```python
from build123d import *

# Parameters (mm, degrees)
F0_W     = 170
F0_H     = 60
F1_DEPTH = 60
F2_R     = 20
F3_T     = -10
F4_SCALE = 1.2


with BuildPart() as f1:
    # F0 (on Top) → F1 (new body, symmetric)
    with BuildSketch(Plane.XY):
        Rectangle(F0_W, F0_H)
    extrude(amount=F1_DEPTH, both=True)

    # F2
    f2_edges = [f1.edges().sort_by_distance(p)[0] for p in [
        (-85, -30, 0),
        (-85, 30, 0),
        (85, -30, 0),
        (85, 30, 0),
        (0, 30, -60),
        (0, -30, -60),
        (-85, 0, -60),
        (85, 0, -60),
    ]]
    fillet(f2_edges, radius=F2_R)

    # F3
    f3_openings = [f1.faces().sort_by_distance(p)[0] for p in [
        (0, 0, 60),
    ]]
    offset(amount=F3_T, openings=f3_openings)


with BuildPart() as f1_1:
    # F4: moved
    add(f1.part.scale(F4_SCALE))


solid = f1_1.part
```
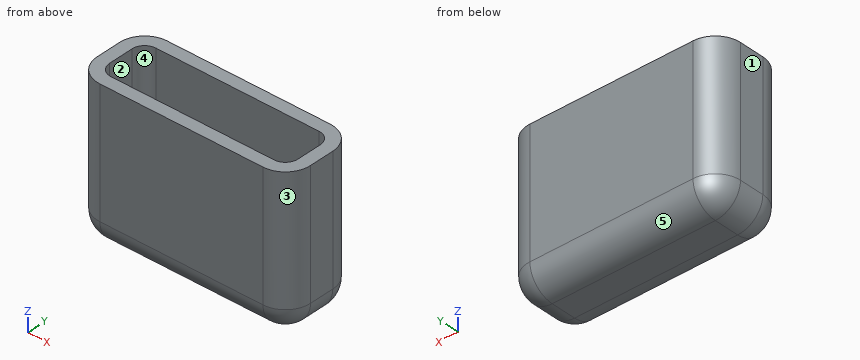
Here's how the part is built. I have some questions about the finished solid (model axes, mm). Face numbers are marked on the shaded views. A direction names the side the tool comes from. Round coordinates to 2 decimals unless told otherwise and drop trailing zeros. Order: outer loops, then holes, each group sorted by start corner. A loop starts at its lowest first (then second) coordinate and runs counter-clockwise, first axis right, second up. Notation, with made-up numbers: (-17, 10.25) -> (8, 10.25) arc R12 ccw to (8, 17.25) -> close; hole circle Ø6 at (13.5, -19). An arc over 180 degrees is marked (long way). Use a Markdown table: item, result. Add a question column.
(1) Suppose I cut it at A-A, the plane z = -2.5. Please give me the cut outline in (x, y).
(2) If we mould it in two halves opening along Y, with no side actions, what happens to the marked faces 1, 2 and 3? For each: released by +Y, released by -Y, zero draft, split by the parting line, or undercut.
(3) I need wall thicknesses on line 1 along Y through (x, z) = (56, -7); line 2 along X through (y, z) = (9, -22); line 3 along Z through (x, y) = (16, 1). Which ranges of each line are inside material? Lowest first, please.
(4) Suppose I cut it at D-D, the plane y = -31. Please give me the cut outline in (x, z).
(5) Suppose I cut it at C-C, the plane x = -2. Please give me the cut outline in (y, z).
(6) For pin 1 Ø4 at (x, y) = (-57.5, 15) entering from +Z; pin 2 Ø10 at (x, z) = (-66, -55) entering from +Y; pin 3 Ø4 at (x, y) = (30.5, 10.5) entering from +Z, each with a flat end and sliding along its axis, tell me the tip position at first contact or that it passes through.
(7) For the marked faces 4 and 5, which set-ups out of +Z, -Z, +X, -X, +Y, -Y let a thin tool reach every point of the face, with its end or its side?
(8) Suppose I cut it at B-B, the plane y = -3. Please give me the cut outline in (x, z).
Verdict:
| question | item | result |
|---|---|---|
| 1 | outline | (-102, -12) arc R24 ccw to (-78, -36) -> (78, -36) arc R24 ccw to (102, -12) -> (102, 12) arc R24 ccw to (78, 36) -> (-78, 36) arc R24 ccw to (-102, 12) -> close; hole (-90, -12) arc R12 ccw to (-78, -24) -> (78, -24) arc R12 ccw to (90, -12) -> (90, 12) arc R12 ccw to (78, 24) -> (-78, 24) arc R12 ccw to (-90, 12) -> close |
| 2 | face 1 | zero draft |
| 2 | face 2 | undercut |
| 2 | face 3 | released by -Y |
| 3 | line 1 | -36 to -24, 24 to 36 |
| 3 | line 2 | -102 to -90, 90 to 102 |
| 3 | line 3 | -72 to -60 |
| 4 | outline | (-92.66, -48) arc R14.66 ccw to (-78, -62.66) -> (78, -62.66) arc R14.66 ccw to (92.66, -48) -> (92.66, 72) -> (-92.66, 72) -> close |
| 5 | outline | (-36, -48) arc R24 ccw to (-12, -72) -> (12, -72) arc R24 ccw to (36, -48) -> (36, 72) -> (24, 72) -> (24, -48) arc R12 cw to (12, -60) -> (-12, -60) arc R12 cw to (-24, -48) -> (-24, 72) -> (-36, 72) -> close |
| 6 | pin 1 | z = -58.91 |
| 6 | pin 2 | y = 35.92 |
| 6 | pin 3 | z = -59.99 |
| 7 | face 4 | +Z |
| 7 | face 5 | -Z, +X, -X, +Y |
| 8 | outline | (-102, -48) arc R24 ccw to (-78, -72) -> (78, -72) arc R24 ccw to (102, -48) -> (102, 72) -> (90, 72) -> (90, -48) arc R12 cw to (78, -60) -> (-78, -60) arc R12 cw to (-90, -48) -> (-90, 72) -> (-102, 72) -> close |
